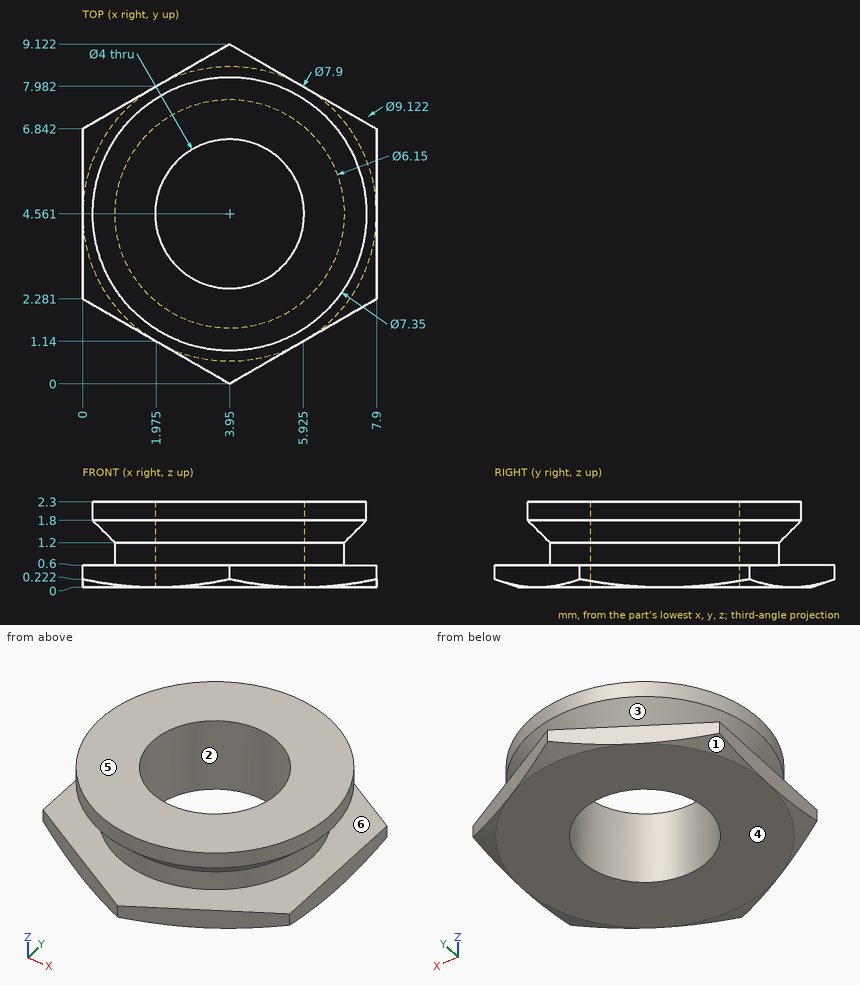
Print and shaded views of the part. All mm, measured from the part's lowest x, y and z. A direction names the side the tool comes from. Round coordinates to 2 decimals unless told otherwise and drop trailing zeros. Use CSV: the item, a comma, the result in double quotes. Start each with the question number.
1) Pull direction Y, two halves, no side cores. Call the marked faces 1, 2, 3 and 4: +Y half, -Y half, draft (parallel to the pull), parting line (faces both ways), or undercut.
2) Drop a flat-ended pin along its axis: P1, Ø3.5, axis at x = 3.95, y = 4.56, coming from the +Z side. Give the stop position or say it passes through.
3) Wall check: L1, parallel to X at y = 3.75, z = 0.5; L2, parallel to Y at x = 5.5, z = 0.25 (1 decimal); L3, parallel to X at y = 3.25, z = 1.6. Give the ranges that are in metal, low to high. Write a range as [from, to].
4) Which spindle directions (+Z, -Z, +X, -X, +Y, -Y) get a long thin tool onto all of the face, cutting with end or side? Do the marked faces 5 and 6. Say none if no direction does.
Determined:
1,face 1,"+Y half"
1,face 2,"undercut"
1,face 3,"parting line"
1,face 4,"draft"
2,P1,"passes through"
3,L1,"x = [0, 2.12], [5.78, 7.9]"
3,L2,"y = [0.9, 3.3], [5.8, 8.2]"
3,L3,"x = [0.73, 2.44], [5.46, 7.17]"
4,face 5,"+Z, +X, -X, +Y, -Y"
4,face 6,"none"
